from build123d import *

# Parameters (mm, degrees)
SKETCH1_R           = 1.6
BOSS_EXTRUDE1_DEPTH = 3
SKETCH2_W           = 19.6
SKETCH2_H           = 3
BOSS_EXTRUDE2_DEPTH = 40


with BuildPart() as part:
    # Sketch1 → Boss-Extrude1 (new body)
    with BuildSketch(Plane.XZ.offset(561.298939869)):
        Polygon((-11.110843614, 789.420141885), (16.239156386, 789.420141885), (16.239156386, 739.620141885), (86.639156386, 739.620141885), (86.639156386, 789.420141885), (105.589156386, 789.420141885), (105.589156386, 545.720141885), (-31.210843614, 545.720141885), (-31.210843614, 727.020141885), (-11.110843614, 727.020141885), align=None)
        with Locations((-21.210843614, 703.620141885)):
            Circle(SKETCH1_R, mode=Mode.SUBTRACT)
        with Locations((-21.210843614, 587.620141885)):
            Circle(SKETCH1_R, mode=Mode.SUBTRACT)
    extrude(amount=BOSS_EXTRUDE1_DEPTH)

    # Sketch2 → Boss-Extrude2 (add)
    with BuildSketch(Plane.ZY.offset(11.110843614)):
        with Locations((779.620141885, -562.798939869)):
            Rectangle(SKETCH2_W, SKETCH2_H)
    extrude(amount=BOSS_EXTRUDE2_DEPTH)


solid = part.part
CAD build for the part. Positions are in the model's coordinates, mm. Round coordinates to 2 decimals unless told otherwise and drop trailing zeros. Write each loop counter-clockwise with the first axis right and the second up, starting at its lowest first coordinate (ties: lowest second). Pieces come first, ordered by that corner, then holes. Notation, with made-up numbers: M 3.5,17.5 L 27.5,17.5 A20 ccw 27.5,52.5 Z; hole C 65,-13.5 d11. An arc over 180 degrees is marked long. Put each result on its own line as item: value. Start each with the question number.
1) Drill centre lines: probe 1 along Z at (x, y) = (-21, -563.1); probe 2 along Z at (x, y) = (-20, -562.6); probe 3 along Z at (x, y) = (86, -563.6). Where is each one in solid material? Low to high. Write a range as [from, to].
2) Pin check, flat tips, straight feed: pin 1 Ø1.5 at (y, z) = (-562.5, 633.5) entering from -X; pin 2 Ø0.9 at (x, y) = (50.5, -563.5) entering from +Z; pin 3 Ø5 at (x, z) = (-21.21, 703.62) entering from +Y; pin 4 Ø2.5 at (x, z) = (-21.21, 587.62) entering from -Y. Stop position of each tip, or through.
3) Saw through at D-D, the plane x = 65.5. Write the cut outline in (y, z).
4) Saw through at A-A, the plane x = -28. Write the cut outline in (y, z), and give its area (3 significant figures).
5) Saw through at C-C, the plane y = -563.3. Write the cut outline in (x, z), and give its area (3 significant figures).
6) Saw through at B-B, the plane z = 760. Write the cut outline in (x, y).
Resolved:
1. probe 1: [545.72, 586.03], [589.21, 702.03], [705.21, 727.02], [769.82, 789.42]
1. probe 2: [545.72, 586.57], [588.67, 702.57], [704.67, 727.02], [769.82, 789.42]
1. probe 3: [545.72, 739.62]
2. pin 1: x = -31.21
2. pin 2: z = 739.62
2. pin 3: y = -561.3
2. pin 4: through
3. outline: M -564.3,545.72 L -561.3,545.72 L -561.3,739.62 L -564.3,739.62 Z
4. outline: M -564.3,545.72 L -561.3,545.72 L -561.3,727.02 L -564.3,727.02 Z; M -564.3,769.82 L -561.3,769.82 L -561.3,789.42 L -564.3,789.42 Z
4. area: 603 mm²
5. outline: M -51.11,769.82 L -11.11,769.82 L -11.11,727.02 L -31.21,727.02 L -31.21,545.72 L 105.59,545.72 L 105.59,789.42 L 86.64,789.42 L 86.64,739.62 L 16.24,739.62 L 16.24,789.42 L -51.11,789.42 Z; hole C -21.21,587.62 d3.2; hole C -21.21,703.62 d3.2
5. area: 29,300 mm²
6. outline: M -11.11,-564.3 L 16.24,-564.3 L 16.24,-561.3 L -11.11,-561.3 Z; M 86.64,-564.3 L 105.59,-564.3 L 105.59,-561.3 L 86.64,-561.3 Z
